Design review of the part built by this model. Coordinates are the model's own, in mm. Coordinates: 2 decimals unless noted, no trailing zeros. Write each loop counter-clockwise with the first axis right and the second up, starting at its lowest first coordinate (ties: lowest second). Pieces come first, ordered by that corner, then holes.
```python
from build123d import *

# Parameters (mm, degrees)
PAD_DEPTH           = 20
FILLET_R            = 1
SKETCH001_R         = 2
POCKET_DEPTH        = 20.001
LINEARPATTERN_COUNT = 6
LINEARPATTERN_PITCH = 7.2
FILLET001_R         = 2


with BuildPart() as part:
    # Sketch → Pad (new body)
    with BuildSketch(Plane.XY):
        Polygon((0, 0), (50, 0), (50, -12), align=None)
    extrude(amount=PAD_DEPTH)

    # Fillet
    fillet_edges = [part.edges().sort_by_distance(p)[0] for p in [
        (0, 0, 10),
    ]]
    fillet(fillet_edges, radius=FILLET_R)

    # Sketch001 (on Face5 of Fillet) → Pocket (cut, through all)
    with BuildSketch(Plane.XY.offset(20)):
        with Locations((47, 0)):
            Circle(SKETCH001_R)
    pocket = extrude(amount=-POCKET_DEPTH, mode=Mode.SUBTRACT)

    # LinearPattern: Pocket ×6
    with Locations(*[(-i * LINEARPATTERN_PITCH, 0, 0) for i in range(1, LINEARPATTERN_COUNT)]):
        add(pocket, mode=Mode.SUBTRACT)

    # Fillet001
    fillet001_edges = [part.edges().sort_by_distance(p)[0] for p in [
        (13, 0, 10),
        (16.2, 0, 10),
        (20.2, 0, 10),
        (23.4, 0, 10),
        (27.4, 0, 10),
        (30.6, 0, 10),
        (34.6, 0, 10),
        (37.8, 0, 10),
        (41.8, 0, 10),
        (45, 0, 10),
    ]]
    fillet(fillet001_edges, radius=FILLET001_R)


solid = part.part
```
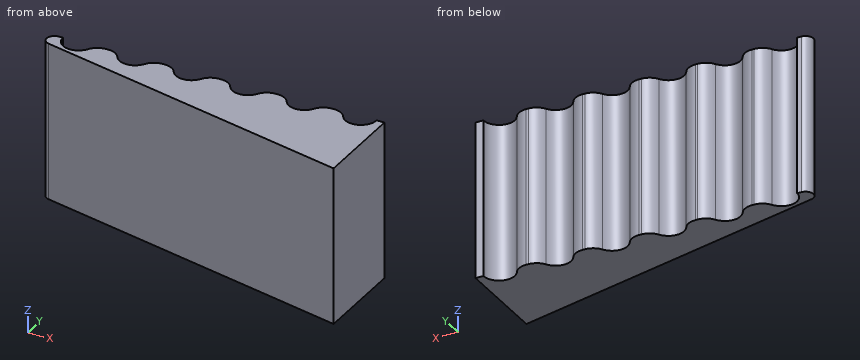
(1) Wall thickness on line 1 (Y direction, x = 43.5, z = 5); line 2 (Y direction, x = 42, z = 12.5): over which ranges is each line inside the solid? List them lowest first.
(2) Consider section C-C (x = 40.5). Give the boundary of the cut face in (y, z), plus the area to 3 significant figures.
(3) Insertion check: pin 1 Ø2 at (x, z) = (26, 7) entering from +Y; pin 2 Ø10 at (x, z) = (35, 8) entering from +Y. Each pin has a flat end and moves straight along its axis. Give the tip position at first contact, or say it passes through.
(4) Consider section B-B (y = -6). Give the boundary of the cut face in (x, z), plus the area to 3 significant figures.
(5) Consider section A-A (z = 8.5). Give the boundary of the cut face in (x, y), plus the area to 3 significant figures.
Results:
1. line 1: y = -10.44 to 0
1. line 2: y = -10.08 to -0.45
2. outline: (-9.72, 0) - (-1.87, 0) - (-1.87, 20) - (-9.72, 20) - close
2. area: 157 mm2
3. pin 1: stops at y = -1.2
3. pin 2: stops at y = 0
4. outline: (25, 0) - (50, 0) - (50, 20) - (25, 20) - close
4. area: 500 mm2
5. outline: (8.22, -1.97) - (50, -12) - (50, 0) - (49, 0) arc R2 cw to (45.27, -1) arc R2 ccw to (43.54, 0) - (43.26, 0) arc R2 ccw to (41.53, -1) arc R2 cw to (38.07, -1) arc R2 ccw to (36.34, 0) - (36.06, 0) arc R2 ccw to (34.33, -1) arc R2 cw to (30.87, -1) arc R2 ccw to (29.14, 0) - (28.86, 0) arc R2 ccw to (27.13, -1) arc R2 cw to (23.67, -1) arc R2 ccw to (21.94, 0) - (21.66, 0) arc R2 ccw to (19.93, -1) arc R2 cw to (16.47, -1) arc R2 ccw to (14.74, 0) - (14.46, 0) arc R2 ccw to (12.73, -1) arc R2 cw to (9, 0) - (8.45, 0) arc R1 ccw to start
5. area: 252 mm2
